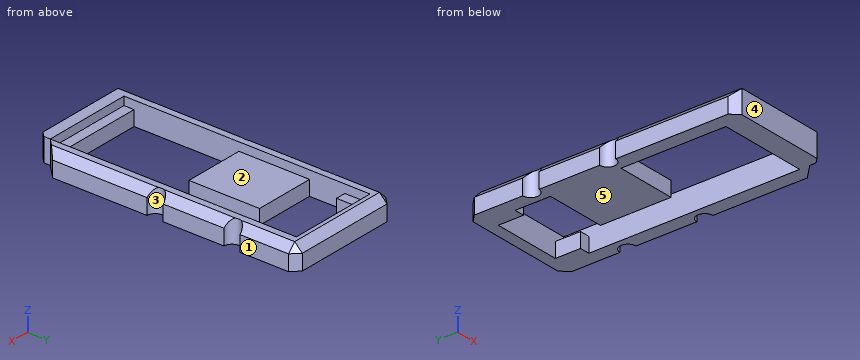
from build123d import *

# Parameters (mm, degrees)
SKETCH_W        = 23.32
SKETCH_H        = 53.34
PAD_DEPTH       = 4.6
SKETCH001_W     = 17.68
SKETCH001_H     = 48.8
POCKET_DEPTH    = 1.65
POCKET001_DEPTH = 3
SKETCH003_R     = 1.6
POCKET002_DEPTH = 5
CHAMFER_SIZE    = 1.5
POCKET003_DEPTH = 5
CHAMFER001_SIZE = 1


with BuildPart() as part:
    # Sketch → Pad (new body)
    with BuildSketch(Plane.XY):
        with Locations((11.66, 26.67)):
            Rectangle(SKETCH_W, SKETCH_H)
    extrude(amount=PAD_DEPTH)

    # Sketch001 (on Face6 of Pad) → Pocket (cut)
    with BuildSketch(Plane.XY.offset(4.6)):
        with Locations((11.66, 26.67)):
            Rectangle(SKETCH001_W, SKETCH001_H)
    extrude(amount=-POCKET_DEPTH, mode=Mode.SUBTRACT)

    # Sketch002 (on Face11 of Pocket) → Pocket001 (cut)
    with BuildSketch(Plane.XY.offset(2.95)):
        Polygon((2.82, 4.27), (20.5, 4.27), (20.5, 46.07), (18.5, 46.07), (18.5, 51.07), (4.82, 51.07), (4.82, 46.07), (2.82, 46.07), (2.82, 39.07), (14.82, 39.07), (14.82, 25.07), (2.82, 25.07), align=None)
    extrude(amount=-POCKET001_DEPTH, mode=Mode.SUBTRACT)

    # Sketch003 (on Face5 of Pocket001) → Pocket002 (cut)
    with BuildSketch(Plane.XY.offset(4.6)):
        with Locations((23.32, 40.64)):
            Circle(SKETCH003_R)
        with Locations((23.32, 25.4)):
            Circle(SKETCH003_R)
        with Locations((0, 40.64)):
            Circle(SKETCH003_R)
        with Locations((0, 25.4)):
            Circle(SKETCH003_R)
    extrude(amount=-POCKET002_DEPTH, mode=Mode.SUBTRACT)

    # Chamfer
    chamfer_edges = [part.edges().sort_by_distance(p)[0] for p in [
        (23.32, 47.79, 4.6),
        (11.66, 53.34, 4.6),
        (0, 47.79, 4.6),
        (0, 33.02, 4.6),
        (23.32, 33.02, 4.6),
        (23.32, 11.9, 4.6),
        (0, 11.9, 4.6),
        (23.32, 0, 2.3),
        (0, 0, 2.3),
        (23.32, 53.34, 2.3),
        (0, 53.34, 2.3),
    ]]
    chamfer(chamfer_edges, length=CHAMFER_SIZE)

    # Sketch004 (on Face35 of Chamfer) → Pocket003 (cut)
    with BuildSketch(Plane.XY.offset(4.6)):
        Polygon((24.23, 6), (24.23, 0), (20.5, 0), (20.5, 2.27), align=None)
    extrude(amount=-POCKET003_DEPTH, mode=Mode.SUBTRACT)

    # Chamfer001
    chamfer001_edges = [part.edges().sort_by_distance(p)[0] for p in [
        (20.5, 0, 2.3),
    ]]
    chamfer(chamfer001_edges, length=CHAMFER001_SIZE)


solid = part.part
The model under review builds one solid part; all positions refer to its coordinate system, in mm. Face numbers are marked on the shaded views. A direction names the side the tool comes from. Give positions to 0.01 mm unless a question says otherwise; leave off trailing zeros. Loops run counter-clockwise (first coordinate to the right, second up) from the corner with the lowest first, then second, coordinate; pieces in that order, holes last. Notation, with made-up numbers: (-26, -37.75) -> (6, -37.75) arc R20 ccw to (6, -27.75) -> close; hole circle Ø4 at (34.5, -4.75). An arc over 180 degrees is marked (long way). Answer as a JSON object with one key per item and string values. Group by question number.
Q1. Insertion check: pin 1 (1 mm diameter, centred on x = 10.5, y = 3, fed in from +Z); pin 2 (10 mm diameter, centred on x = 9.5, y = 21.5, fed in from -Z); pin 3 (0.5 mm diameter, centred on x = 15, z = 4, fed in from +Y). Each pin has a flat end and moves straight along its axis. Give the tip position at first contact, or say it passes through.
Q2. Draft analysis for pull direction Y (two halves, no side actions). For the marked faces 3, 4 and 5, state which applies: pulls with the +Y half, pulls with the -Y half, needs draft (parallel to the pull), parting line crosses it, or undercut.
Q3. Take a section at B-B (x = 6.25). Write out the cut boundary in (y, z).
Q4. Take a section at A-A (y = 29). Write out the cut boundary in (x, z).
Q5. Tool access review of the marked faces 1 and 2: name each direction out of +Z, -Z, +X, -X, +Y, -Y from which nothing blocks a thin tool from reaching the whole face with its end or side.
Q6. Take a section at D-D (y = 40.64). Write out the cut boundary in (x, z), plus the area to 3 significant figures.
Q7. Wall thickness on line 1 along Y through (x, z) = (6.5, 0.8); line 2 along Y through (x, z) = (4.75, 0.95); line 3 along X through (y, z) = (45, 2.5): over which ranges is each line inside the solid? List them lowest first.
Answer below:
{
 "1": {"pin 1": "stops at z = 2.95", "pin 2": "stops at z = 0", "pin 3": "stops at y = 52.69"},
 "2": {"face 3": "undercut", "face 4": "pulls with the -Y half", "face 5": "needs draft"},
 "3": {"outline": "(0, 0) -> (4.27, 0) -> (4.27, 2.95) -> (2.27, 2.95) -> (2.27, 4.6) -> (0, 4.6) -> close; (25.07, 0) -> (39.07, 0) -> (39.07, 2.95) -> (25.07, 2.95) -> close; (51.07, 0) -> (53.34, 0) -> (53.34, 3.1) -> (51.84, 4.6) -> (51.07, 4.6) -> close"},
 "4": {"outline": "(0, 0) -> (14.82, 0) -> (14.82, 2.95) -> (2.82, 2.95) -> (2.82, 4.6) -> (1.5, 4.6) -> (0, 3.1) -> close; (20.5, 0) -> (23.32, 0) -> (23.32, 3.1) -> (21.82, 4.6) -> (20.5, 4.6) -> close"},
 "5": {"face 1": "+Z, -Z, +X, +Y, -Y", "face 2": "+Z"},
 "6": {"outline": "(1.6, 0) -> (2.82, 0) -> (2.82, 4.6) -> (1.6, 4.6) -> close; (20.5, 0) -> (21.72, 0) -> (21.72, 4.6) -> (20.5, 4.6) -> close", "area": "11.2 mm2"},
 "7": {"line 1": "y = 0 to 4.27, 25.07 to 39.07, 51.07 to 53.34", "line 2": "y = 0 to 4.27, 25.07 to 39.07, 46.07 to 53.34", "line 3": "x = 0 to 2.82, 20.5 to 23.32"}
}
